Source: three-view drawing plus pictorial views. Frame: mm from the lowest corner of the part. A direction names the side the tool comes from. Coordinates: 2 decimals unless noted, no trailing zeros. Order: outer loops, then holes, each group sorted by start corner. A loop starts at its lowest first (then second) coordinate and runs counter-clockwise, first axis right, second up. Notation, with made-up numbers: M -39.75,88.25 L -23.75,88.25 A21 ccw -23.75,123.25 Z; hole C 6,58.25 d9. An arc over 180 degrees is marked long. Use CSV: the item, a comma, the result in double quotes. Start each with the question number.
Q1. Section query C-C, the plane y = 3.75. Output: boundary loops of the cut face in (x, z), and give its area (3 significant figures).
Q2. Ray query, probe 1 along Z at (x, y) = (63.5, 13.75); probe 2 along Y at (x, z) = (68.58, 0.55) (1 decimal); probe 3 along Z at (x, y) = (5, 8.25). Return the intervals inside material, ascending.
Q3. Access query for the marked faces 5 and 6. Directions: +Z, -Z, +X, -X, +Y, -Y. A direction counts if a zero-diameter tool reaches every point of the face in a straight line with its end or side. Return the directions, or none.
Q4. Section query D-D, the plane x = 21. Output: boundary loops of the cut face in (y, z), and give its area (3 significant figures).
Q5. Section query A-A, the plane y = 9.5. Output: boundary loops of the cut face in (x, z) (1 decimal).
Q6. Mould query, pull axis Z, two halves, no side actions, for the marked faces 1, 2, 3 and 4. Classes: +Z half, -Z half, draft (parallel to the pull), parting line (faces both ways), or undercut.
Q7. Section query B-B, the plane x = 7.62. Output: boundary loops of the cut face in (y, z) (1 decimal).
Q8. First-contact query: P1, Ø4, axis at x = 68.58, y = 9.5, coming from the -Z side; P2, Ø5.5, axis at x = 65.9, y = 15.88, coming from the +Z side; P3, Ø1.5, axis at x = 61, z = 21.5, coming from the +Y side; P4, Ø6, axis at y = 6.5, z = 19, coming from the -X side. Flat tips, straight axial feed; report the tip coordinate or a pass-through.
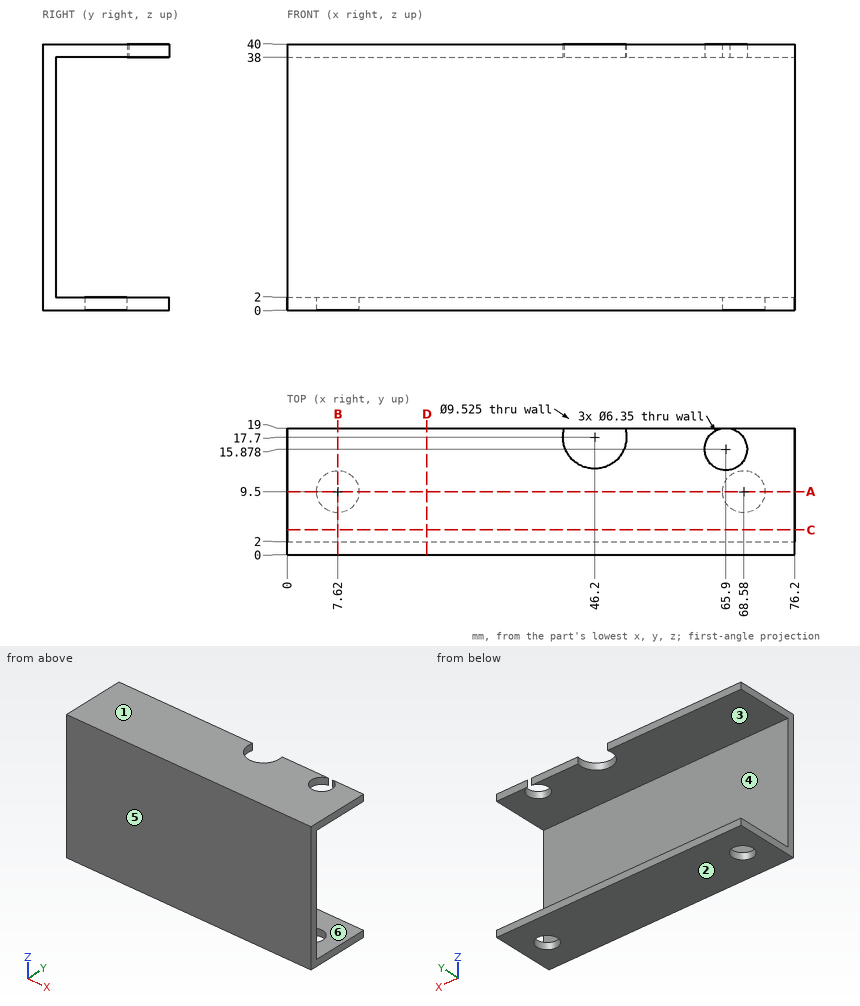
Responses:
1,outline,"M 0,0 L 76.2,0 L 76.2,2 L 0,2 Z; M 0,38 L 76.2,38 L 76.2,40 L 0,40 Z"
1,area,"305 mm²"
2,probe 1,"z = 0 to 2, 38 to 40"
2,probe 2,"y = 0 to 6.3, 12.7 to 19"
2,probe 3,"z = 38 to 40"
3,face 5,"+Z, -Z, +X, -X, -Y"
3,face 6,"+X, -X, +Y"
4,outline,"M 0,0 L 19,0 L 19,2 L 2,2 L 2,38 L 19,38 L 19,40 L 0,40 Z"
4,area,"148 mm²"
5,outline,"M 0,0 L 4.4,0 L 4.4,2 L 0,2 Z; M 0,38 L 76.2,38 L 76.2,40 L 0,40 Z; M 10.8,0 L 65.4,0 L 65.4,2 L 10.8,2 Z; M 71.8,0 L 76.2,0 L 76.2,2 L 71.8,2 Z"
6,face 1,"+Z half"
6,face 2,"-Z half"
6,face 3,"undercut"
6,face 4,"undercut"
7,outline,"M 0,0 L 6.3,0 L 6.3,2 L 2,2 L 2,38 L 19,38 L 19,40 L 0,40 Z; M 12.7,0 L 19,0 L 19,2 L 12.7,2 Z"
8,P1,"stops at z = 38"
8,P2,"stops at z = 2"
8,P3,"stops at y = 2"
8,P4,"passes through"
